Geometry check sheet. Reference: the model listing, model coordinates, mm. A direction names the side the tool comes from. Give positions to 0.01 mm unless a question says otherwise; leave off trailing zeros. Order: outer loops, then holes, each group sorted by start corner. A loop starts at its lowest first (then second) coordinate and runs counter-clockwise, first axis right, second up. Notation, with made-up numbers: M 5.5,-37 L 55.5,-37 A22 cw 55.5,-28 Z; hole C 37,85 d6. An arc over 180 degrees is marked long. Answer as CSV lines item,"result".
from build123d import *

# Parameters (mm, degrees)
BOSS_EXTRUDE1_DEPTH     = 7.5
SKETCH2_R               = 3.25
CUT_EXTRUDE1_DEPTH      = 112.91626334
FILLET1_R               = 2
SKETCH3_R               = 2.5
CUT_EXTRUDE2_DEPTH      = 103.592641062
CUT_EXTRUDE4_DEPTH      = 121.158229015
BOSS_EXTRUDE2_REACH     = 128.857
SKETCH7_W               = 5
SKETCH7_H               = 15
FILLET2_R               = 3
SKETCH8_R               = 4.25
CUT_EXTRUDE6_DEPTH      = 4.829629131
CUT_EXTRUDE3_DEPTH      = 125.202455692
CUT_EXTRUDE3_DEPTH_BACK = 125.202455692
SKETCH4_W               = 50
SKETCH4_H               = 7
CHAMFER1_START          = -7.5
CHAMFER1_DEPTH          = 15
CHAMFER2_SIZE           = 5


with BuildPart() as part:
    # Sketch1 → Boss-Extrude1 (new, symmetric)
    with BuildSketch(Plane.XY):
        Polygon((-28, 13), (-113, 13), (-113, 38), (-103, 38), (-103, 23), (-88, 23), (-88, 27), (-28, 27), (-28, 22.5), (-8, 22.5), (-8, -22.5), (-28, -22.5), (-28, -27), (-88, -27), (-88, -23), (-103, -23), (-103, -38), (-113, -38), (-113, -13), (-28, -13), (-16, -9.784609691), (-16, 9.784609691), align=None)
    extrude(amount=BOSS_EXTRUDE1_DEPTH, both=True)

    # Sketch2 → Cut-Extrude1 (cut, through all)
    with BuildSketch(Plane(origin=(-8, 0, 0), x_dir=(0, 0, -1), z_dir=(1, 0, 0))):
        Circle(SKETCH2_R)
    extrude(amount=-CUT_EXTRUDE1_DEPTH, mode=Mode.SUBTRACT)

    # Fillet1
    fillet1_edges = [part.edges().sort_by_distance(p)[0] for p in [
        (-103, -23, 0),
        (-103, 23, 0),
    ]]
    fillet(fillet1_edges, radius=FILLET1_R)

    # Sketch3 → Cut-Extrude2 (cut, through all)
    with BuildSketch(Plane(origin=(-103, 0, 0), x_dir=(0, 0, -1), z_dir=(1, 0, 0))):
        with Locations((0, 33.5)):
            Circle(SKETCH3_R)
        with Locations((0, -33)):
            Circle(SKETCH3_R)
    extrude(amount=-CUT_EXTRUDE2_DEPTH, mode=Mode.SUBTRACT)

    # Sketch5 → Cut-Extrude4 (cut, through all)
    with BuildSketch(Plane.XY.offset(7.5)):
        with BuildLine():
            Line((-77.5, 23.000000001), (-32.5, 23.000000001))
            ThreePointArc((-32.5, 23.000000001), (-31.5, 22.000000001), (-32.5, 21.000000001))
            Line((-32.5, 21.000000001), (-77.5, 21.000000001))
            ThreePointArc((-77.5, 21.000000001), (-78.5, 22.000000001), (-77.5, 23.000000001))
        make_face()
        with BuildLine():
            Line((-77.5, -23.000000001), (-32.5, -23.000000001))
            ThreePointArc((-32.5, -23.000000001), (-31.5, -22.000000001), (-32.5, -21.000000001))
            Line((-32.5, -21.000000001), (-77.5, -21.000000001))
            ThreePointArc((-77.5, -21.000000001), (-78.5, -22.000000001), (-77.5, -23.000000001))
        make_face()
    extrude(amount=-CUT_EXTRUDE4_DEPTH, mode=Mode.SUBTRACT)

    # Boss-Extrude2: up to this plane
    boss_extrude2_end = Plane(origin=(-16, -9.784609691, -7.5), z_dir=(-0.25881904510251796, 0.9659258262890691, 0))
    # Sketch7 → Boss-Extrude2 (add, up to the surface)
    with BuildSketch(Plane(origin=(1.374355653, 5.129165125, 0), x_dir=(-0.9659258262890691, 0.25881904510251813, 0), z_dir=(-0.25881904510251813, -0.9659258262890691, 0)), mode=Mode.PRIVATE) as boss_extrude2_sk1:
        with Locations((25.021910533, 0)):
            Rectangle(SKETCH7_W, SKETCH7_H)
    boss_extrude2_tool1 = split(extrude(boss_extrude2_sk1.sketch, amount=BOSS_EXTRUDE2_REACH, dir=(0, -1, 0), mode=Mode.PRIVATE), bisect_by=boss_extrude2_end, keep=Keep.BOTH, mode=Mode.PRIVATE)
    add(boss_extrude2_tool1.solids().sort_by_distance((-22.794954, 11.605312, 0))[0])

    # Fillet2
    fillet2_edges = [part.edges().sort_by_distance(p)[0] for p in [
        (-20.380139389, -10.958264503, 0),
        (-20.380139389, 10.958264503, 0),
        (-88, -23, 0),
        (-88, 23, 0),
    ]]
    fillet(fillet2_edges, radius=FILLET2_R)

    # Sketch8 → Cut-Extrude6 (cut)
    with BuildSketch(Plane.ZY.offset(25.20976852)):
        with Locations(Location((0, 0, 0), (0, 0, 270))):
            Circle(SKETCH8_R)
    extrude(amount=-CUT_EXTRUDE6_DEPTH, mode=Mode.SUBTRACT)

    # Sketch4 → Cut-Extrude3 (cut, two sides: drawn at the far end of the back side and taken through both)
    with BuildSketch(Plane(origin=(0, 13, 0), x_dir=(-1, 0, 0), z_dir=(0, -1, 0)).offset(-CUT_EXTRUDE3_DEPTH_BACK)):
        with Locations((50.20976852, 0)):
            Rectangle(SKETCH4_W, SKETCH4_H)
    extrude(amount=CUT_EXTRUDE3_DEPTH + CUT_EXTRUDE3_DEPTH_BACK, mode=Mode.SUBTRACT)

    # Chamfer1: read off the stored shape, not the designer's step
    # Chamfer1 outline → Chamfer1 (cut)
    with BuildSketch(Plane.XY.offset(CHAMFER1_START)):
        Polygon((-28, 27), (-33, 27), (-28.5, 22.5), (-28, 22.5), align=None)
        with BuildLine():
            Line((-88.401923788, 24.5), (-84.07179677, 27))
            Line((-84.07179677, 27), (-88, 27))
            Line((-88, 27), (-88, 26))
            ThreePointArc((-88, 26), (-88.102222521, 25.223542864), (-88.401923788, 24.5))
        make_face()
        Polygon((-28.5, -22.5), (-33, -27), (-28, -27), (-28, -22.5), align=None)
        with BuildLine():
            Line((-84.07179677, -27), (-88.401923788, -24.5))
            ThreePointArc((-88.401923788, -24.5), (-88.102222521, -25.223542864), (-88, -26))
            Line((-88, -26), (-88, -27))
            Line((-88, -27), (-84.07179677, -27))
        make_face()
    extrude(amount=CHAMFER1_DEPTH, mode=Mode.SUBTRACT)

    # Chamfer2
    chamfer2_edges = [part.edges().sort_by_distance(p)[0] for p in [
        (-8, 22.5, 0),
        (-8, -22.5, 0),
    ]]
    chamfer(chamfer2_edges, length=CHAMFER2_SIZE)


solid = part.part
(1) Tool access check on faces 1 (the face through (-78.5, -22, 0.1)), 2 (the face through (-65, 27, 5)), 3 (the face through (-75.21, 25, 0)). Record the directions out of +Z, -Z, +X, -X, +Y, -Y that give a thin tool (end or side, any length) a straight path to the whole face; none if there is none.
The answers:
face 1,"+Z, -Z"
face 2,"+Z, -Z, +X, +Y"
face 3,"+X, +Y, -Y"
(2) Draft check along Z on faces 4 (the face through (-26.585, 12.621, -5.472)), 5 (the face through (-50, 20, 3.5)). Enter one of: +Z half, -Z half, draft (parallel to the pull), parting line (faces both ways), or undercut.
The answers:
face 4,"draft"
face 5,"undercut"
(3) Gauge pin test, flat ends, axial feed: P1, Ø8, axis at x = -87, z = 4.5, coming from the -Y side; P2, Ø6, axis at x = -29.5, z = -3.5, coming from the +Y side; P3, Ø1.2, axis at y = -24.5, z = -0.5, coming from the +X side. Record the tip position at first contact, or that the pin passes through.
The answers:
P1,"stops at y = -27"
P2,"stops at y = 26.5"
P3,"stops at x = -75.21"
(4) Material ranges on line 1 (Y direction, x = -58.5, z = -4.5); line 2 (Y direction, x = -106.25, z = 0); line 3 (Y direction, x = -13, z = 0), recorded low to high.
The answers:
line 1,"y = -27 to -23, -21 to -13, 13 to 21, 23 to 27"
line 2,"y = -38 to -35.5, -30.5 to -13, 13 to 31, 36 to 38"
line 3,"y = -22.5 to -3.25, 3.25 to 22.5"
(5) Section check A-A on x = -63.5. State how many separate pieces and enclosed holes the cut face has, then the cut area to 3 significant figures.
The answers:
separate pieces,"8"
enclosed holes,"0"
area,"192 mm2"
(6) Section check B-B on y = -33. Enter the section's corners in (x, z), then the cut area to 3 significant figures.
The answers:
outline,"M -113,-7.5 L -103,-7.5 L -103,-2.5 L -113,-2.5 Z; M -113,2.5 L -103,2.5 L -103,7.5 L -113,7.5 Z"
area,"100 mm2"
